from build123d import *

# Parameters (mm, degrees)
F1_DEPTH = 4
F3_DEPTH = 2
F4_R     = 1.5
F5_DEPTH = 4.001


with BuildPart() as f1:
    # F0 (on Right) → F1 (new body)
    with BuildSketch(Plane.YZ):
        with BuildLine():
            Line((48.14, 18.44), (-1.027172, 3.345881))
            ThreePointArc((-1.027172, 3.345881), (-3.462092, -0.513727), (-0.011339, -3.499982))
            Line((-0.011339, -3.499982), (49.38, -3.66))
            Line((49.38, -3.66), (84.37, 16.43))
            Line((84.37, 16.43), (84.24, 21.35))
            Line((84.24, 21.35), (48.14, 18.44))
        make_face()
    extrude(amount=F1_DEPTH)

    # F2 (on face) → F3 (cut)
    with BuildSketch(Plane.YZ.offset(4)):
        with BuildLine():
            ThreePointArc((46.75, 5.163873), (44.23, 8.88), (46.75, 12.596127))
            ThreePointArc((46.75, 12.596127), (47.207647, 12.96391), (47.38, 13.525159))
            Line((47.38, 13.525159), (47.38, 14.7615))
            ThreePointArc((47.38, 14.7615), (46.974358, 15.565701), (46.086522, 15.717466))
            Line((46.086522, 15.717466), (3.834993, 2.746421))
            ThreePointArc((3.834993, 2.746421), (3.220284, 2.20902), (3.211033, 1.392576))
            ThreePointArc((3.211033, 1.392576), (3.462092, 0.513727), (3.47705, -0.400156))
            ThreePointArc((3.47705, -0.400156), (3.722981, -1.178735), (4.467253, -1.514481))
            Line((4.467253, -1.514481), (46.37676, -1.65026))
            ThreePointArc((46.37676, -1.65026), (47.08596, -1.358516), (47.38, -0.650265))
            Line((47.38, -0.650265), (47.38, 4.234841))
            ThreePointArc((47.38, 4.234841), (47.207647, 4.79609), (46.75, 5.163873))
        make_face()
        with BuildLine():
            Line((49.38, 15.610834), (49.38, 13.394144))
            ThreePointArc((49.38, 13.394144), (49.534423, 12.860291), (49.95, 12.491316))
            ThreePointArc((49.95, 12.491316), (52.21832, 8.574543), (49.38, 5.048877))
            Line((49.38, 5.048877), (49.38, 0.373496))
            ThreePointArc((49.38, 0.373496), (49.878964, -0.49193), (50.877926, -0.493723))
            Line((50.877926, -0.493723), (81.846475, 17.287304))
            Line((81.846475, 17.287304), (81.797347, 19.146612))
            Line((81.797347, 19.146612), (50.299651, 16.607601))
            ThreePointArc((50.299651, 16.607601), (49.645034, 16.288938), (49.38, 15.610834))
        make_face()
    extrude(amount=-F3_DEPTH, mode=Mode.SUBTRACT)

    # F4 (on face) → F5 (cut, through all)
    with BuildSketch(Plane.YZ.offset(4)):
        Circle(F4_R)
        with Locations((48.23, 8.88)):
            Circle(F4_R)
    extrude(amount=-F5_DEPTH, mode=Mode.SUBTRACT)


solid = f1.part
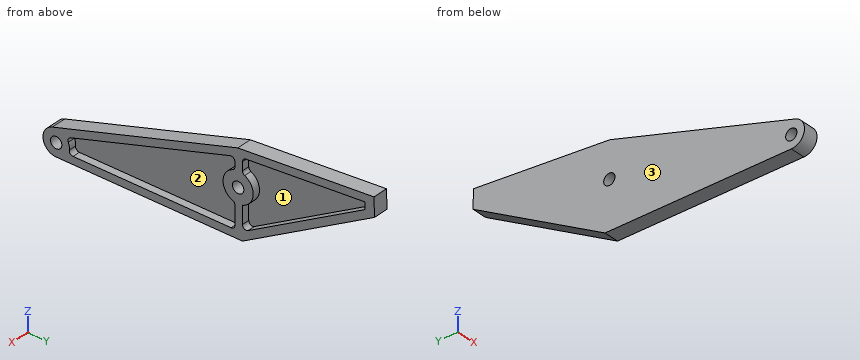
Geometry check sheet. Reference: the model listing, model coordinates, mm. Face numbers are marked on the shaded views. Give positions to 0.01 mm unless a question says otherwise; leave off trailing zeros. Write each loop counter-clockwise with the first axis right and the second up, starting at its lowest first coordinate (ties: lowest second). Pieces come first, ordered by that corner, then holes. Notation, with made-up numbers: M 29,-5.75 L 81,-5.75 A22 cw 81,32.25 Z; hole C 60.5,-11 d7. An arc over 180 degrees is marked long. One line per question, with ' | ' between items.
1. Scan lines: line 1 along Z through (x, y) = (1.2, 48.23); line 2 along X through (y, z) = (37.5, 11); line 3 along Z through (x, y) = (0.5, 49). Record each from-to range of solid material in increasing order. Write a range as from..to.
Ans:
line 1: -3.66..7.38, 10.38..18.45 | line 2: 0..2 | line 3: -3.66..7.59, 10.17..18.51
2. Cross-section at B-B (z = 8.88). Enter the section's corners in (x, y).
Ans:
outline: M 0,17 L 4,17 L 4,23.81 L 2,23.81 L 2,44.23 L 4,44.23 L 4,46.73 L 0,46.73 Z; M 0,49.73 L 4,49.73 L 4,52.23 L 2,52.23 L 2,67.2 L 4,67.2 L 4,71.22 L 0,71.22 Z
3. Cross-section at A-A (x = 1.35). Enter the section's corners in (y, z).
Ans:
outline: M -1.03,3.35 A3.5 ccw -0.01,-3.5 L 49.38,-3.66 L 84.37,16.43 L 84.24,21.35 L 48.14,18.44 Z; hole C 0,0 d3; hole C 48.23,8.88 d3
4. Gauge pin test, flat ends, axial feed: pin 1 (2 mm diameter, centred on x = 1, y = 21.5, fed in from +Z); pin 2 (1.6 mm diameter, centred on x = 2.5, z = 2.5, fed in from -Y); pin 3 (2 mm diameter, centred on x = 2.5, z = 2, fed in from +Y). Record the tip position at first contact, or that the pin passes through.
Ans:
pin 1: z = 10.57 | pin 2: y = -3.06 | pin 3: y = 60.98
5. Mould release check, pull along Z, two halves, no side actions. Record for the marked faces 1, 2 and 3: released by +Z, released by -Z, zero draft, split by the parting line, or undercut.
Ans:
face 1: undercut | face 2: undercut | face 3: zero draft
6. Cross-section at C-C (y = 7). Enter the section's corners in (x, z), plus the area to 4 significant figures.
Ans:
outline: M 0,-3.52 L 4,-3.52 L 4,-1.52 L 2,-1.52 L 2,3.72 L 4,3.72 L 4,5.81 L 0,5.81 Z | area: 26.85 mm2
7. Cross-section at D-D (y = 34.5). Enter the section's corners in (x, z), plus the area to 3 significant figures.
Ans:
outline: M 0,-3.61 L 4,-3.61 L 4,-1.61 L 2,-1.61 L 2,12.16 L 4,12.16 L 4,14.25 L 0,14.25 Z | area: 43.9 mm2
